Input: part model. Units: mm. Frame: model coordinates. A direction names the side the tool comes from. Give positions to 0.01 mm unless a question says otherwise; leave off trailing zeros. Loops run counter-clockwise (first coordinate to the right, second up) from the corner with the lowest first, then second, coordinate; pieces in that order, holes last.
from build123d import *

# Parameters (mm, degrees)
SKETCH_1_R               = 42.7
EXTRUDE_1_DEPTH          = 5
SKETCH_2_R               = 42.7
SKETCH_2_R_2             = 35
EXTRUDE_2_DEPTH          = 6
SKETCH_3_R               = 1.5
CUT_EXTRUDE_1_DEPTH      = 11
SKETCH_4_R               = 6
CUT_EXTRUDE_2_DEPTH      = 11
CUT_EXTRUDE_3_DEPTH      = 11
SKETCH_6_R               = 10
CUT_EXTRUDE_4_DEPTH      = 11
CUT_EXTRUDE_START        = -6
CUT_EXTRUDE_5_DEPTH      = 6
CUT_EXTRUDE_6_DEPTH      = 50
CUT_EXTRUDE_6_DEPTH_BACK = 50
SKETCH_9_R               = 1.5
CUT_EXTRUDE_7_DEPTH      = 50
CUT_EXTRUDE_7_DEPTH_BACK = 50
SKETCH_10_R              = 1.5
EXTRUDE_12_DEPTH         = 36
EXTRUDE_12_DEPTH_BACK    = 36
SKETCH_13_R              = 1.5
EXTRUDE_13_DEPTH         = 36
EXTRUDE_13_DEPTH_BACK    = 36
SKETCH_14_R              = 1.5
SKETCH_15_R              = 35
CUT_EXTRUDE_8_DEPTH      = 6
SKETCH_16_R              = 10
CUT_EXTRUDE_9_DEPTH      = 6
SKETCH_17_R              = 1.5
CUT_EXTRUDE_11_DEPTH     = 1.1
CUT_EXTRUDE_START_2      = -1.1
SKETCH_18_R              = 1.5
CUT_EXTRUDE_12_DEPTH     = 1.1
SKETCH_19_R              = 1.5
CUT_EXTRUDE_13_DEPTH     = 1.1
SKETCH_20_R              = 1.5
CUT_EXTRUDE_14_DEPTH     = 1.1
SKETCH_21_R              = 6
CUT_EXTRUDE_15_DEPTH     = 5


with BuildPart() as part:
    # Sketch 1 → Extrude 1 (new body)
    with BuildSketch(Plane.XY):
        Circle(SKETCH_1_R)
    extrude(amount=EXTRUDE_1_DEPTH)

    # Sketch 2 → Extrude 2 (add)
    with BuildSketch(Plane.XY.offset(5)):
        Circle(SKETCH_2_R)
        Circle(SKETCH_2_R_2, mode=Mode.SUBTRACT)
    extrude(amount=EXTRUDE_2_DEPTH)

    # Sketch 3 → Cut-Extrude 1 (cut)
    with BuildSketch(Plane.XY.offset(11)):
        with Locations((0, 39)):
            Circle(SKETCH_3_R)
        with Locations((39, 0)):
            Circle(SKETCH_3_R)
        with Locations((0, -39)):
            Circle(SKETCH_3_R)
        with Locations((-39, 0)):
            Circle(SKETCH_3_R)
    extrude(amount=-CUT_EXTRUDE_1_DEPTH, mode=Mode.SUBTRACT)

    # Sketch 4 → Cut-Extrude 2 (cut)
    with BuildSketch(Plane.XY.offset(11)):
        with Locations((0, 29)):
            Circle(SKETCH_4_R)
        with Locations((-29, 0)):
            Circle(SKETCH_4_R)
        with Locations((0, -29)):
            Circle(SKETCH_4_R)
        with Locations((29, 0)):
            Circle(SKETCH_4_R)
    extrude(amount=-CUT_EXTRUDE_2_DEPTH, mode=Mode.SUBTRACT)

    # Sketch 5 → Cut-Extrude 3 (cut)
    with BuildSketch(Plane.XY.offset(5)):
        with BuildLine():
            ThreePointArc((30.612068966, 13.607028833), (23.68807717, 23.68807717), (13.607028833, 30.612068966))
            ThreePointArc((13.607028833, 30.612068966), (7.667150024, 28.327809843), (9.951409146, 22.387931034))
            ThreePointArc((9.951409146, 22.387931034), (17.324116139, 17.324116139), (22.387931034, 9.951409146))
            ThreePointArc((22.387931034, 9.951409146), (28.327809843, 7.667150024), (30.612068966, 13.607028833))
        make_face()
        with BuildLine():
            ThreePointArc((-13.607028833, 30.612068966), (-23.68807717, 23.68807717), (-30.612068966, 13.607028833))
            ThreePointArc((-30.612068966, 13.607028833), (-28.327809843, 7.667150024), (-22.387931034, 9.951409146))
            ThreePointArc((-22.387931034, 9.951409146), (-17.324116139, 17.324116139), (-9.951409146, 22.387931034))
            ThreePointArc((-9.951409146, 22.387931034), (-7.667150024, 28.327809843), (-13.607028833, 30.612068966))
        make_face()
    extrude(amount=-CUT_EXTRUDE_3_DEPTH, mode=Mode.SUBTRACT)

    # Sketch 6 → Cut-Extrude 4 (cut)
    with BuildSketch(Plane.XY.offset(5)):
        Circle(SKETCH_6_R)
    extrude(amount=-CUT_EXTRUDE_4_DEPTH, mode=Mode.SUBTRACT)

    # Sketch 7 → Cut-Extrude 5 (cut)
    with BuildSketch(Plane.XY.offset(11).offset(CUT_EXTRUDE_START)):
        with BuildLine():
            Line((-14.251220498, 31.967213115), (-17.386489007, 39))
            ThreePointArc((-17.386489007, 39), (-30.193459557, 30.193459557), (-39, 17.386489007))
            Line((-39, 17.386489007), (-31.967213115, 14.251220498))
            ThreePointArc((-31.967213115, 14.251220498), (-24.748737342, 24.748737342), (-14.251220498, 31.967213115))
        make_face()
        with BuildLine():
            ThreePointArc((39.206540603, 16.915589672), (30.374710616, 30.011113858), (17.386489007, 39))
            Line((17.386489007, 39), (14.251220498, 31.967213115))
            ThreePointArc((14.251220498, 31.967213115), (24.897303783, 24.599273654), (32.136508691, 13.865237436))
            Line((32.136508691, 13.865237436), (39.206540603, 16.915589672))
        make_face()
        with BuildLine():
            ThreePointArc((17.386489007, -39), (30.006036038, -30.379726814), (38.78183243, -17.867833483))
            Line((38.78183243, -17.867833483), (31.788387238, -14.64576515))
            ThreePointArc((31.788387238, -14.64576515), (24.595111506, -24.901415422), (14.251220498, -31.967213115))
            Line((14.251220498, -31.967213115), (17.386489007, -39))
        make_face()
        with BuildLine():
            Line((-31.967213115, -14.251220498), (-39, -17.386489007))
            ThreePointArc((-39, -17.386489007), (-30.193459557, -30.193459557), (-17.386489007, -39))
            Line((-17.386489007, -39), (-14.251220498, -31.967213115))
            ThreePointArc((-14.251220498, -31.967213115), (-24.748737342, -24.748737342), (-31.967213115, -14.251220498))
        make_face()
    extrude(amount=CUT_EXTRUDE_5_DEPTH, mode=Mode.SUBTRACT)

    # Sketch 9 → Cut-Extrude 6 (cut, two sides: drawn at the far end of the back side and taken through both)
    with BuildSketch(Plane(origin=(0, 0, 0), x_dir=(0, 0, -1), z_dir=(-0.2079116908177632, -0.9781476007338048, 0)).offset(-CUT_EXTRUDE_6_DEPTH_BACK)):
        with Locations(Location((-5.905553742, 0, 0), (0, 0, 270))):
            Circle(SKETCH_9_R)
    extrude(amount=CUT_EXTRUDE_6_DEPTH + CUT_EXTRUDE_6_DEPTH_BACK, mode=Mode.SUBTRACT)

    # Sketch 10 → Cut-Extrude 7 (cut, two sides: drawn at the far end of the back side and taken through both)
    with BuildSketch(Plane(origin=(0, 0, 0), x_dir=(0, 0, -1), z_dir=(0.9781476007338056, -0.2079116908177598, 0)).offset(-CUT_EXTRUDE_7_DEPTH_BACK)):
        with Locations(Location((-5.905553742, 0, 0), (0, 0, 270))):
            Circle(SKETCH_10_R)
    extrude(amount=CUT_EXTRUDE_7_DEPTH + CUT_EXTRUDE_7_DEPTH_BACK, mode=Mode.SUBTRACT)

    # Sketch 13 → Extrude 12 (add, two sides: drawn at the far end of the back side and taken through both)
    with BuildSketch(Plane(origin=(0, 0, 0), x_dir=(0, 0, -1), z_dir=(-0.2079116908177632, -0.9781476007338048, 0)).offset(-EXTRUDE_12_DEPTH_BACK)):
        with Locations(Location((-5.905553742, 0, 0), (0, 0, 270))):
            Circle(SKETCH_13_R)
    extrude(amount=EXTRUDE_12_DEPTH + EXTRUDE_12_DEPTH_BACK)

    # Sketch 14 → Extrude 13 (add, two sides: drawn at the far end of the back side and taken through both)
    with BuildSketch(Plane(origin=(0, 0, 0), x_dir=(0, 0, -1), z_dir=(0.9781476007338056, -0.2079116908177598, 0)).offset(-EXTRUDE_13_DEPTH_BACK)):
        with Locations(Location((-5.905553742, 0, 0), (0, 0, 270))):
            Circle(SKETCH_14_R)
    extrude(amount=EXTRUDE_13_DEPTH + EXTRUDE_13_DEPTH_BACK)

    # Sketch 15 → Cut-Extrude 8 (cut)
    with BuildSketch(Plane.XY.offset(11).offset(CUT_EXTRUDE_START)):
        Circle(SKETCH_15_R)
    extrude(amount=CUT_EXTRUDE_8_DEPTH, mode=Mode.SUBTRACT)

    # Sketch 16 → Cut-Extrude 9 (cut)
    with BuildSketch(Plane.XY.offset(5)):
        Circle(SKETCH_16_R)
    extrude(amount=-CUT_EXTRUDE_9_DEPTH, mode=Mode.SUBTRACT)

    # Sketch 17 → Cut-Extrude 11 (cut)
    with BuildSketch(Plane(origin=(35.213313626, -7.484820869, 0), x_dir=(0, 0, -1), z_dir=(0.9781476007338056, -0.2079116908177598, 0))):
        with Locations(Location((-5.905553742, 0, 0), (0, 0, 270))):
            Circle(SKETCH_17_R)
    extrude(amount=-CUT_EXTRUDE_11_DEPTH, mode=Mode.SUBTRACT)

    # Sketch 18 → Cut-Extrude 12 (cut)
    with BuildSketch(Plane(origin=(-35.213313626, 7.484820869, 0), x_dir=(0, 0, 1), z_dir=(-0.9781476007338056, 0.2079116908177598, 0)).offset(CUT_EXTRUDE_START_2)):
        with Locations(Location((5.905553742, 0, 0), (0, 0, 270))):
            Circle(SKETCH_18_R)
    extrude(amount=CUT_EXTRUDE_12_DEPTH, mode=Mode.SUBTRACT)

    # Sketch 19 → Cut-Extrude 13 (cut)
    with BuildSketch(Plane(origin=(7.484820869, 35.213313626, 0), x_dir=(0.9781476007338048, -0.2079116908177632, 0), z_dir=(0.2079116908177632, 0.9781476007338048, 0))):
        with Locations(Location((0, -5.905553742, 0), (0, 0, 180))):
            Circle(SKETCH_19_R)
    extrude(amount=-CUT_EXTRUDE_13_DEPTH, mode=Mode.SUBTRACT)

    # Sketch 20 → Cut-Extrude 14 (cut)
    with BuildSketch(Plane(origin=(-7.484820869, -35.213313626, 0), x_dir=(0.9781476007338048, -0.2079116908177632, 0), z_dir=(-0.2079116908177632, -0.9781476007338048, 0)).offset(CUT_EXTRUDE_START_2)):
        with Locations(Location((0, 5.905553742, 0), (0, 0, 180))):
            Circle(SKETCH_20_R)
    extrude(amount=CUT_EXTRUDE_14_DEPTH, mode=Mode.SUBTRACT)

    # Sketch 21 → Cut-Extrude 15 (cut)
    with BuildSketch(Plane.XY.offset(5)):
        with Locations((0, 29)):
            Circle(SKETCH_21_R)
        with Locations((-29, 0)):
            Circle(SKETCH_21_R)
        with Locations((0, -29)):
            Circle(SKETCH_21_R)
        with Locations((29, 0)):
            Circle(SKETCH_21_R)
    extrude(amount=-CUT_EXTRUDE_15_DEPTH, mode=Mode.SUBTRACT)


solid = part.part
(1) Reachability of faces 1 (the flat face through (37, 0, 11)), 2 (the flat face through (-35.434, -15.797, 7.958)), 3 (the cylindrical face through (0, 35, 8)), 4 (the cylindrical face through (-17.413, 17.235, 2.535)), 5 (the flat face through (-15.84, -35.53, 7.96)) from +Z, -Z, +X, -X, +Y, -Y: full face, straight path, thin tool, end or side. Return the list, or none.
Values follow:
face 1: +Z, +X, -X, +Y, -Y
face 2: +Z, -Y
face 3: +Z
face 4: +Z, -Z
face 5: +Z, -X
(2) Pin query (flat end, axial travel): pin 1 Ø1 at (y, z) = (17, 4) entering from +X; pin 2 Ø4 at (x, y) = (-22, -10) entering from +Z; pin 3 Ø9.5 at (x, y) = (0, 29) entering from +Z; pin 4 Ø1 at (y, z) = (21, 1.5) entering from -X. Return the tip coordinate at first contact, or that it passes through.
Values follow:
pin 1: stops at x = 39.38
pin 2: stops at z = 5
pin 3: passes through
pin 4: stops at x = -37.46
(3) Cut plane C-C (x = -29.5). Return the cut outline in (y, z), and give its area (3 significant figures).
Values follow:
outline: (-30.87, 0) - (-5.98, 0) - (-5.98, 5) - (-30.87, 5) - close; (5.98, 0) - (8.43, 0) - (8.43, 5) - (5.98, 5) - close; (15.87, 0) - (30.87, 0) - (30.87, 5) - (15.87, 5) - close
area: 212 mm2
(4) Ray query, probe 1 along Y at (x, z) = (0, 3.75); probe 2 along Y at (x, z) = (-29, 3.95); probe 3 along Y at (x, z) = (0, 8.75). Return the intervals inside material, ascending.
Values follow:
probe 1: y = -42.7 to -40.5, -37.5 to -35, -23 to -10, 10 to 23, 35 to 37.5, 40.5 to 42.7
probe 2: y = -31.34 to -6, 6 to 8.04, 16.77 to 31.34
probe 3: y = -42.7 to -40.5, -37.5 to -35, 35 to 37.5, 40.5 to 42.7
(5) Mould query, pull axis X, two halves, no side actions, for faces 6 (the flat face through (-35.53, 15.84, 7.96)), 7 (the flat face through (0, -37, 11)), 8 (the flat face through (15.797, -35.434, 7.958)). Classes: +X half, -X half, draft (parallel to the pull), parting line (faces both ways), or undercut.
Values follow:
face 6: undercut
face 7: draft
face 8: +X half
(6) Cut plane D-D (y = 26.5). Return the cut outline in (x, z).
Values follow:
outline: (-33.48, 0) - (-20.49, 0) - (-20.49, 5) - (-33.48, 5) - close; (-7.28, 0) - (-5.45, 0) - (-5.45, 5) - (-7.28, 5) - close; (5.45, 0) - (7.28, 0) - (7.28, 5) - (5.45, 5) - close; (20.49, 0) - (33.48, 0) - (33.48, 5) - (20.49, 5) - close
(7) Cut plane A-A (z = 2). Count the separate pieces of the cut face and the enclosed holes in it, and give its area (3 significant figures).
Values follow:
separate pieces: 1
enclosed holes: 11
area: 4,420 mm2
(8) Cut plane B-B (y = -29). Return the cut outline in (x, z), and give its area (3 significant figures).
Values follow:
outline: (-31.34, 0) - (-6, 0) - (-6, 5) - (-31.34, 5) - close; (6, 0) - (31.34, 0) - (31.34, 5) - (6, 5) - close
area: 253 mm2
